The listing builds one solid part. Answer for the finished solid, in the listing's coordinates (mm). Coordinates: 2 decimals unless noted, no trailing zeros. Loops run counter-clockwise (first coordinate to the right, second up) from the corner with the lowest first, then second, coordinate; pieces in that order, holes last. Notation, with made-up numbers: (-22.5, 59) - (-5.5, 59) arc R21 ccw to (-5.5, 63) - close; hole circle Ø1 at (29.5, 80). An arc over 180 degrees is marked (long way). Put each result on its own line as item: value.
```python
from build123d import *

# Parameters (mm, degrees)
SKETCH1_R               = 0.5
EXTRUDE1_DEPTH          = 45
SHELL1_T                = -0.1
CUT_EXTRUDE1_DEPTH      = 45
CUT_EXTRUDE1_DEPTH_BACK = 45


with BuildPart() as part:
    # Sketch1 → Extrude1 (new body)
    with BuildSketch(Plane(origin=(0, 0, 0), x_dir=(1, 0, 0), z_dir=(0, 1, 0))):
        with Locations(Location((0, 0, 0), (0, 0, 270))):
            Circle(SKETCH1_R)
    extrude(amount=EXTRUDE1_DEPTH)

    # Shell1
    shell1_openings = [part.faces().sort_by_distance(p)[0] for p in [
        (0, 45, 0),
        (0, 0, 0),
    ]]
    offset(amount=SHELL1_T, openings=shell1_openings, kind=Kind.INTERSECTION)

    # Sketch2 → Cut-Extrude1 (cut, two sides: drawn at the far end of the back side and taken through both)
    with BuildSketch(Plane.XY.offset(-CUT_EXTRUDE1_DEPTH_BACK)):
        Polygon((-0.5, 45), (3.966783564, 39.557315291), (3.966783564, 46.045953815), align=None)
    extrude(amount=CUT_EXTRUDE1_DEPTH + CUT_EXTRUDE1_DEPTH_BACK, mode=Mode.SUBTRACT)


solid = part.part
```
1) The part is cut by section A-A (x = -0.2). Give the vertices of the cut face in (y, z), and give its area (3 significant figures).
Found:
outline: (0, -0.46) - (44.63, -0.46) - (44.63, -0.35) - (0, -0.35) - close; (0, 0.35) - (44.63, 0.35) - (44.63, 0.46) - (0, 0.46) - close
area: 9.98 mm^2
2) The part is cut by section C-C (y = 27). Give the vertices of the cut face in (x, z).
Found:
outline: circle Ø1 at (0, 0); hole circle Ø0.8 at (0, 0)
3) The part is cut by section B-B (z = 0). Give the vertices of the cut face in (x, y), and give its area (3 significant figures).
Found:
outline: (-0.5, 0) - (-0.4, 0) - (-0.4, 44.88) - (-0.5, 45) - close; (0.4, 0) - (0.5, 0) - (0.5, 43.78) - (0.4, 43.9) - close
area: 8.88 mm^2
4) Straight lines are drawn through the part: L1, parallel to X at y = 28, z = -0.35; L2, parallel to Y at x = -0.35, z = -0.3. For each, find the intervals that lie inside material, in ascending order. Write a range as [from, to].
Found:
L1: x = [-0.36, -0.19], [0.19, 0.36]
L2: y = [0, 44.82]
